Part model, mm, in its own coordinate system. Round coordinates to 2 decimals unless told otherwise and drop trailing zeros. Loops run counter-clockwise (first coordinate to the right, second up) from the corner with the lowest first, then second, coordinate; pieces in that order, holes last. Notation, with made-up numbers: M 18.5,70 L 54.5,70 A8 ccw 54.5,74 Z; hole C -11.75,-33 d1. An arc over 180 degrees is marked long. Put each result on its own line as item: value. Start each with the question number.
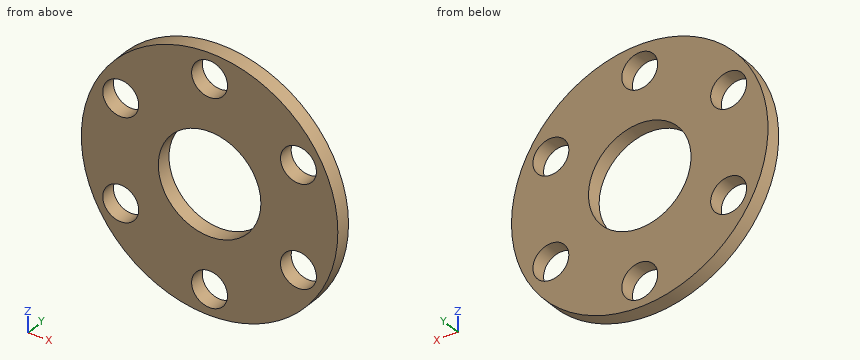
```python
from build123d import *

# Parameters (mm, degrees)
SKETCH1_R           = 12.5
SKETCH1_R_2         = 5
BOSS_EXTRUDE1_DEPTH = 1.5
SKETCH2_R           = 1.75
CUT_EXTRUDE1_DEPTH  = 2.5
CIRPATTERN1_COUNT   = 6


with BuildPart() as part:
    # Sketch1 → Boss-Extrude1 (new body)
    with BuildSketch(Plane(origin=(0, 0, 0), x_dir=(1, 0, 0), z_dir=(0, 1, 0))):
        Circle(SKETCH1_R)
        Circle(SKETCH1_R_2, mode=Mode.SUBTRACT)
    extrude(amount=BOSS_EXTRUDE1_DEPTH)

    # Sketch2 → Cut-Extrude1 (cut, through all)
    with BuildSketch(Plane(origin=(0, 0, 0), x_dir=(1, 0, 0), z_dir=(0, 1, 0))):
        with Locations((0, 10)):
            Circle(SKETCH2_R)
    cut_extrude1 = extrude(amount=CUT_EXTRUDE1_DEPTH, mode=Mode.SUBTRACT)

    # CirPattern1: Cut-Extrude1 ×6 about axis
    cirpattern1_axis = Axis((0, 0, 0), (0, 1, 0))
    for i in range(1, CIRPATTERN1_COUNT):
        add(cut_extrude1.rotate(cirpattern1_axis, i * 360 / CIRPATTERN1_COUNT), mode=Mode.SUBTRACT)


solid = part.part
```
1. Drop a flat-ended pin along its axis: pin 1 (10 mm diameter, centred on x = -0.5, z = -5.5, fed in from -Y). Give the stop position or say it passes through.
2. Wall check: L1, parallel to Z at x = 0, y = 0.4; L2, parallel to Z at x = -10, y = 0.1; L3, parallel to X at y = 0.45, z = -5.75. Give the ranges that are in metal, low to high.
3. Cut at C-C, the plane x = -3. Give the cut face in (y, z), and give its area (3 significant figures).
4. Cut at B-B, the plane x = 10. Give the cut face in (y, z), and give its area (3 significant figures).
5. Cut at D-D, the plane y = 0.9. Give the cut face in (x, z), and give its area (3 significant figures).
6. Cut at A-A, the plane z = -10. Give the cut face in (x, y), and give its area (4 significant figures).
Results list:
1. pin 1: stops at y = 0
2. L1: z = -12.5 to -11.75, -8.25 to -5, 5 to 8.25, 11.75 to 12.5
2. L2: z = -7.5 to -6.13, -3.87 to 3.87, 6.13 to 7.5
2. L3: x = -11.1 to -10.24, -7.08 to 7.08, 10.24 to 11.1
3. outline: M 0,-12.13 L 1.5,-12.13 L 1.5,-4 L 0,-4 Z; M 0,4 L 1.5,4 L 1.5,12.13 L 0,12.13 Z
3. area: 24.4 mm^2
4. outline: M 0,-7.5 L 1.5,-7.5 L 1.5,-6.13 L 0,-6.13 Z; M 0,-3.87 L 1.5,-3.87 L 1.5,3.87 L 0,3.87 Z; M 0,6.13 L 1.5,6.13 L 1.5,7.5 L 0,7.5 Z
4. area: 15.7 mm^2
5. outline: C 0,0 d25; hole C -8.66,-5 d3.5; hole C -8.66,5 d3.5; hole C 0,0 d10; hole C 0,-10 d3.5; hole C 0,10 d3.5; hole C 8.66,-5 d3.5; hole C 8.66,5 d3.5
5. area: 355 mm^2
6. outline: M -7.5,0 L -1.75,0 L -1.75,1.5 L -7.5,1.5 Z; M 1.75,0 L 7.5,0 L 7.5,1.5 L 1.75,1.5 Z
6. area: 17.25 mm^2
